Read the model definition and answer for the solid it produces. Units are mm, in the model's axes. Coordinates: 2 decimals unless noted, no trailing zeros. Order: outer loops, then holes, each group sorted by start corner. A loop starts at its lowest first (then second) coordinate and runs counter-clockwise, first axis right, second up. Notation, with made-up numbers: (40, 79) -> (50, 79) arc R14 cw to (50, 96) -> close; hole circle Ø11 at (-19.5, 31). An arc over 180 degrees is marked (long way). Answer in a Markdown table with one row per item.
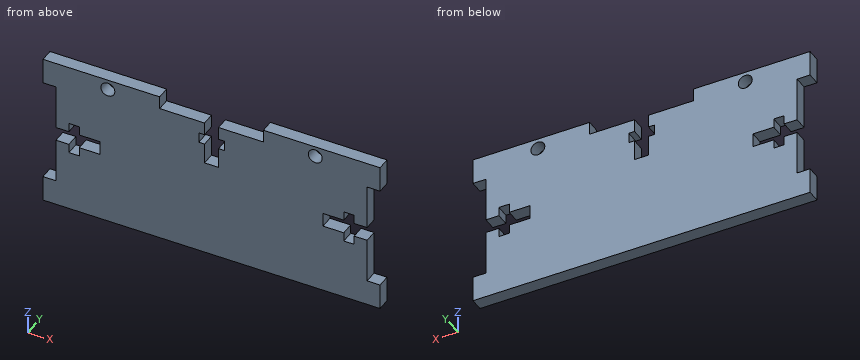
from build123d import *

# Parameters (mm, degrees)
SKETCH1_R           = 1.7145
BOSS_EXTRUDE1_DEPTH = 3.175


with BuildPart() as part:
    # Sketch1 → Boss-Extrude1 (new body)
    with BuildSketch(Plane(origin=(0, 0, 0), x_dir=(1, 0, 0), z_dir=(0, 1, 0))):
        Polygon((-12.7, -3.175), (-12.7, 0), (-1.7145, 0), (-1.7145, 3.175), (-3.120656915, 3.175), (-3.120656915, 5.715), (-1.7145, 5.715), (-1.7145, 10.795), (1.7145, 10.795), (1.7145, 5.715), (3.120656915, 5.715), (3.120656915, 3.175), (1.7145, 3.175), (1.7145, 0), (12.7, 0), (12.7, -3.175), (41.275, -3.175), (41.275, 3.175), (38.1, 3.175), (38.1, 14.1605), (34.925, 14.1605), (34.925, 11.938), (32.385, 11.938), (32.385, 14.1605), (27.305, 14.1605), (27.305, 17.5895), (32.385, 17.5895), (32.385, 19.812), (34.925, 19.812), (34.925, 17.5895), (38.1, 17.5895), (38.1, 28.575), (41.275, 28.575), (41.275, 34.925), (-41.275, 34.925), (-41.275, 28.575), (-38.1, 28.575), (-38.1, 17.5895), (-34.925, 17.5895), (-34.925, 19.812), (-32.385, 19.812), (-32.385, 17.5895), (-27.305, 17.5895), (-27.305, 14.1605), (-32.385, 14.1605), (-32.385, 11.938), (-34.925, 11.938), (-34.925, 14.1605), (-38.1, 14.1605), (-38.1, 3.175), (-41.275, 3.175), (-41.275, -3.175), align=None)
        with Locations(Location((-25.4, -0.635, 0), (0, 0, 270))):
            Circle(SKETCH1_R, mode=Mode.SUBTRACT)
        with Locations(Location((25.4, -0.635, 0), (0, 0, 270))):
            Circle(SKETCH1_R, mode=Mode.SUBTRACT)
    extrude(amount=BOSS_EXTRUDE1_DEPTH)


solid = part.part
Q1. Consider line 1 (X direction, y = 2.4, z = -13.5) (3 decimals); line 2 (Z direction, x = 28, y = 2.2) (1 decimal); line 3 (X direction, y = 1.2, z = -10). Determine where each line is inside the solid, lowest interval first.
Outcome:
| item | result |
|---|---|
| line 1 | -38.1 to -34.925, -32.385 to 32.385, 34.925 to 38.1 |
| line 2 | -34.9 to -17.6, -14.2 to 3.2 |
| line 3 | -38.1 to -1.71, 1.71 to 38.1 |
Q2. The part is cut by section A-A (x = 25.4). Write down the section's boundary in (y, z) (1 decimal), then the cut area to 3 significant figures.
Outcome:
| item | result |
|---|---|
| outline | (0, -34.9) -> (3.2, -34.9) -> (3.2, -1.1) -> (0, -1.1) -> close; (0, 2.3) -> (3.2, 2.3) -> (3.2, 3.2) -> (0, 3.2) -> close |
| area | 110 mm² |
Q3. Given pin 1 (1 mm diameter, centred on x = -9.5, y = 2, fed in from +Z); pin 2 (0.7 mm diameter, centred on y = 1, z = -19, fed in from -X); pin 3 (0.7 mm diameter, centred on y = 2, z = -19, fed in from +X), each flat-ended and moving along its own axis, determine where each tip first touches the part or whether it passes through.
Outcome:
| item | result |
|---|---|
| pin 1 | z = 0 |
| pin 2 | x = -38.1 |
| pin 3 | x = 38.1 |
Q4. The part is cut by section B-B (y = 2). Give the number of separate pieces and of enclosed holes in the cut face, then the cut area to 3 significant figures.
Outcome:
| item | result |
|---|---|
| separate pieces | 1 |
| enclosed holes | 2 |
| area | 2,740 mm² |
Q5. The part is cut by section C-C (x = -8). Write down the section's boundary in (y, z) (3 decimals).
Outcome:
| item | result |
|---|---|
| outline | (0, -34.925) -> (3.175, -34.925) -> (3.175, 0) -> (0, 0) -> close |
